Check sheet for the drawn part. Datum: minimum x, y, z corner. Units: mm. A direction names the side the tool comes from. Coordinates: 2 decimals unless noted, no trailing zeros. Write each loop counter-clockwise with the first axis right and the second up, starting at its lowest first coordinate (ties: lowest second). Pieces come first, ordered by that corner, then holes. Notation, with made-up numbers: (-8.75, 0.25) -> (37.25, 0.25) arc R19 cw to (37.25, 14.25) -> close; hole circle Ø10 at (-24, -17.5). An arc over 180 degrees is marked (long way). Answer in a Markdown table with one row per item. Add a question column.
Q1. Section check C-C, the plane x = 1.25. Record the boundary of the cut face in (y, z), and give its area (3 significant figures).
Q2. Section check A-A, the plane y = 6. Record the boundary of the cut face in (x, z).
Q3. Thickness scan on line 1 (Z direction, x = 1.75, y = 5.25); line 2 (X direction, y = 1.5, z = 0.75); line 3 (Y direction, x = 3.75, z = 5.75). Record the ranges inside material, lowest first.
Q4. Tool access check on the marked faces 1 and 2. Record the directions out of +Z, -Z, +X, -X, +Y, -Y that give a thin tool (end or side, any length) a straight path to the whole face; none if there is none.
Q5. Gauge pin test, flat ends, axial feed: P1, Ø1, axis at x = 3, z = 3.5, coming from the -Y side (3 decimals); P2, Ø2, axis at x = 5, z = 2.5, coming from the -Y side; P3, Ø1.5, axis at x = 3, z = 4.5, coming from the +Y side (3 decimals); P4, Ø3, axis at x = 2, z = 2.5, coming from the -Y side. Record the tip position at first contact, or that the pin passes through.
Q6. Section check D-D, the plane z = 2.5. Record the boundary of the cut face in (x, y) (3 decimals).
Q7. Section check B-B, the plane z = 3.5. Record the boundary of the cut face in (x, y) (3 decimals).
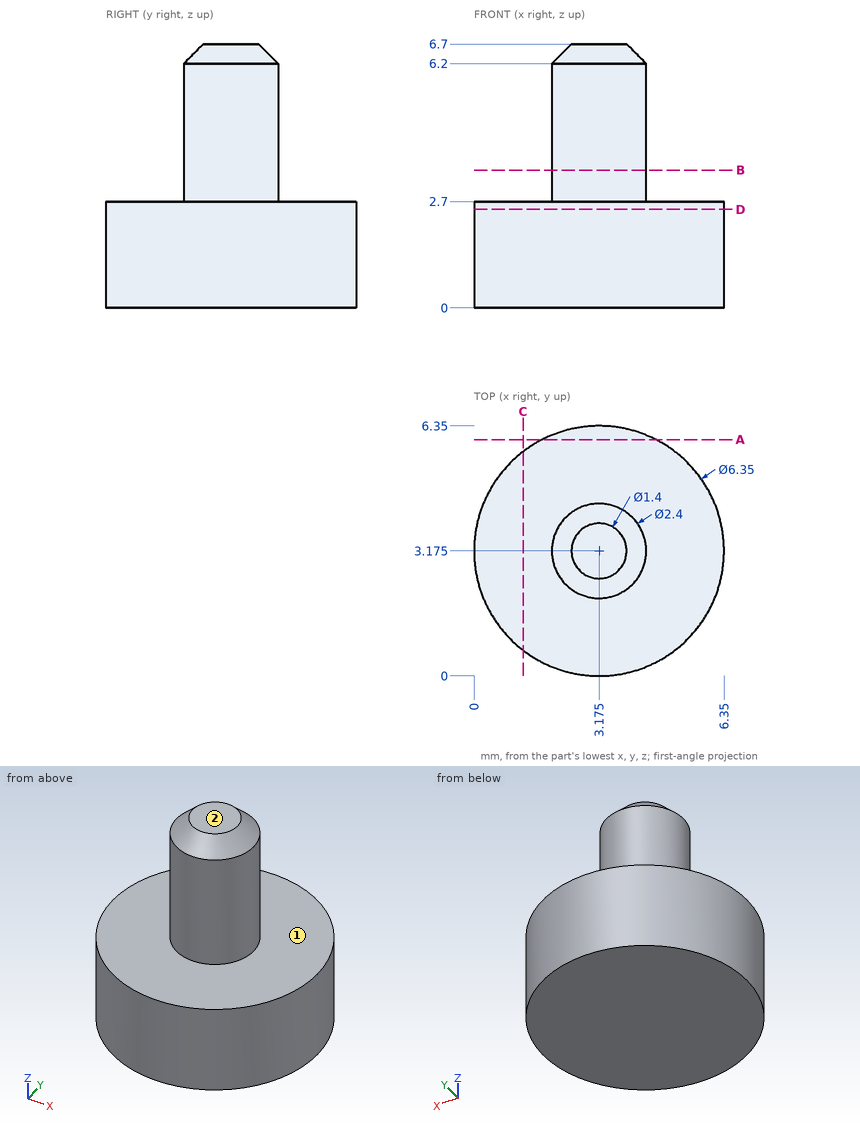
Calculated:
| question | item | result |
|---|---|---|
| 1 | outline | (0.65, 0) -> (5.7, 0) -> (5.7, 2.7) -> (0.65, 2.7) -> close |
| 1 | area | 13.6 mm² |
| 2 | outline | (1.73, 0) -> (4.62, 0) -> (4.62, 2.7) -> (1.73, 2.7) -> close |
| 3 | line 1 | z = 0 to 2.7 |
| 3 | line 2 | x = 0.48 to 5.87 |
| 3 | line 3 | y = 2.12 to 4.23 |
| 4 | face 1 | +Z |
| 4 | face 2 | +Z, +X, -X, +Y, -Y |
| 5 | P1 | stops at y = 1.975 |
| 5 | P2 | stops at y = 0.11 |
| 5 | P3 | stops at y = 4.375 |
| 5 | P4 | stops at y = 0 |
| 6 | outline | circle Ø6.35 at (3.175, 3.175) |
| 7 | outline | circle Ø2.4 at (3.175, 3.175) |
